Geometry check sheet. Reference: the model listing, model coordinates, mm. Face numbers are marked on the shaded views. A direction names the side the tool comes from. Coordinates: 2 decimals unless noted, no trailing zeros. Order: outer loops, then holes, each group sorted by start corner. A loop starts at its lowest first (then second) coordinate and runs counter-clockwise, first axis right, second up. Notation, with made-up numbers: (78, 23.25) -> (116, 23.25) arc R15 cw to (116, 31.25) -> close; hole circle Ø6 at (72.5, 1). An arc over 180 degrees is marked (long way). Answer in a Markdown table with one row per item. Add a question column.
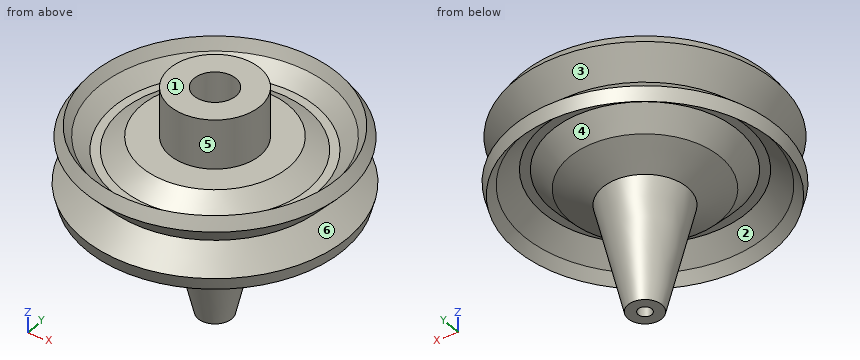
```python
from build123d import *

# Parameters (mm, degrees)
F2_R     = 4.699
F3_DEPTH = 9.398
F4_R     = 1.5367
F5_DEPTH = 17.145


# Not quite as in the source:
# - a feature names something its author has since deleted; it is built from what else it names


with BuildPart() as f1:
    # F0 (on Front) → F1 (revolve)
    with BuildSketch(Plane.XZ):
        Polygon((0, 27.8836265206), (0, -12.487935467), (3.7766563474, -12.487935467), (9.4925444573, 11.6318371147), (16.9307440519, 15.3280049562), (20.9119780944, 19.6802802384), (22.9117851704, 19.6802802384), (27.146894104, 16.1157515753), (28.938142141, 13.8561455533), (29.718, 16.8109368533), (24.366803943, 21.5609171673), (29.371801322, 27.0814523101), (27.6893377921, 29.5746776597), (26.144035833, 27.2886776597), (22.8029862046, 24.1410490125), (20.9119780944, 24.1410490125), (16.4766563474, 27.2050067903), (10.1266563474, 27.2050067903), (10.1266563474, 38.312064533), (0, 38.312064533), align=None)
    revolve(axis=Axis((0, 0, 7.6978455268), (0, 0, -1)))

    # F2 (on face) → F3 (cut)
    with BuildSketch(Plane.XY.offset(38.312064533)):
        Circle(F2_R)
    extrude(amount=-F3_DEPTH, mode=Mode.SUBTRACT)

    # F4 (on face) → F5 (cut)
    with BuildSketch(Plane(origin=(0, 0, -12.487935467), x_dir=(1, 0, 0), z_dir=(0, 0, -1))):
        Circle(F4_R)
    extrude(amount=-F5_DEPTH, mode=Mode.SUBTRACT)


solid = f1.part
```
(1) Go/stop test with flat-tipped pins: P1, Ø5, axis at x = 0, y = 0, coming from the +Z side; P2, Ø4, axis at x = -13, y = 1, coming from the -Z side; P3, Ø1, axis at x = -20, y = -19, coming from the +Z side. Record where each tip stops, or that it passes through.
(2) Access from +Z, -Z, +X, -X, +Y, -Y to the whole of each face (thin tool, end or side, straight path). Record for the marked faces 4, 5 and 6.
(3) Scan lines: line 1 along Y through (x, z) = (0, 36); line 2 along Y through (x, z) = (8, 17); line 3 along X through (y, z) = (5.5, 27.5). Record each from-to range of solid material in increasing order.
(4) Cross-section at C-C (z = -6). Enter the section's corners in (x, y), plus the area to 3 significant figures.
(5) Cross-section at B-B (z = 7). Enter the section's corners in (x, y).
(6) Cross-section at D-D (z = 13). Enter the section's corners in (x, y).
(7) Mould release check, pull along X, two halves, no side actions. Record for the marked faces 1, 2 and 3: +X half, -X half, draft (parallel to the pull), parting line (faces both ways), or undercut.
(8) Cross-section at A-A (z = 33). Enter the section's corners in (x, y), plus the area to 3 significant figures.
Checks:
| question | item | result |
|---|---|---|
| 1 | P1 | z = 28.91 |
| 1 | P2 | z = 12.4 |
| 1 | P3 | z = 29.57 |
| 2 | face 4 | -Z |
| 2 | face 5 | +Z |
| 2 | face 6 | none |
| 3 | line 1 | -10.13 to -4.7, 4.7 to 10.13 |
| 3 | line 2 | -28.4 to -24.84, -16.64 to 16.64, 24.84 to 28.4 |
| 3 | line 3 | -28.56 to -25.71, -8.5 to 8.5, 25.71 to 28.56 |
| 4 | outline | circle Ø10.63 at (0, 0); hole circle Ø3.07 at (0, 0) |
| 4 | area | 81.3 mm² |
| 5 | outline | circle Ø16.79 at (0, 0) |
| 6 | outline | circle Ø24.49 at (0, 0) |
| 7 | face 1 | draft |
| 7 | face 2 | undercut |
| 7 | face 3 | parting line |
| 8 | outline | circle Ø20.25 at (0, 0); hole circle Ø9.4 at (0, 0) |
| 8 | area | 253 mm² |
